Read the model definition and answer for the solid it produces. Units are mm, in the model's axes. Face numbers are marked on the shaded views. A direction names the side the tool comes from. Coordinates: 2 decimals unless noted, no trailing zeros. Loops run counter-clockwise (first coordinate to the right, second up) from the corner with the lowest first, then second, coordinate; pieces in that order, holes last.
from build123d import *

# Parameters (mm, degrees)
BOSS_EXTRUDE1_DEPTH = 7
BOSS_EXTRUDE2_DEPTH = 1
SKETCH3_W           = 57.34
SKETCH3_H           = 7
BOSS_EXTRUDE3_DEPTH = 2
SKETCH4_R           = 2
CUT_EXTRUDE1_DEPTH  = 2


with BuildPart() as part:
    # Sketch1 → Boss-Extrude1 (new body)
    with BuildSketch(Plane.XY):
        Polygon((2, -2), (-55.34, -2), (-55.34, 68.04), (-41.214427125, 68.04), (-38.674427125, 70.58), (-4.251572875, 70.58), (-1.711572875, 68.04), (2, 68.04), align=None)
        Polygon((-53.34, 0), (-53.34, 66.04), (-40.386, 66.04), (-37.846, 68.58), (-5.08, 68.58), (-2.54, 66.04), (0, 66.04), (0, 0), align=None, mode=Mode.SUBTRACT)
    extrude(amount=-BOSS_EXTRUDE1_DEPTH)

    # Sketch2 → Boss-Extrude2 (add)
    with BuildSketch(Plane(origin=(0, 0, -7), x_dir=(-1, 0, 0), z_dir=(0, 0, -1))):
        Polygon((53.34, 0), (0, 0), (0, 66.04), (2.54, 66.04), (5.08, 68.58), (37.846, 68.58), (40.386, 66.04), (53.34, 66.04), align=None)
    extrude(amount=-BOSS_EXTRUDE2_DEPTH)

    # Sketch3 → Boss-Extrude3 (add)
    with BuildSketch(Plane(origin=(0, 0, -7), x_dir=(-1, 0, 0), z_dir=(0, 0, -1))):
        with Locations((26.67, -5.5)):
            Rectangle(SKETCH3_W, SKETCH3_H)
    extrude(amount=-BOSS_EXTRUDE3_DEPTH)

    # Sketch4 → Cut-Extrude1 (cut)
    with BuildSketch(Plane.XY.offset(-5)):
        with Locations((-2.67, -5.5)):
            Circle(SKETCH4_R)
        with Locations((-50.67, -5.5)):
            Circle(SKETCH4_R)
    extrude(amount=-CUT_EXTRUDE1_DEPTH, mode=Mode.SUBTRACT)


solid = part.part
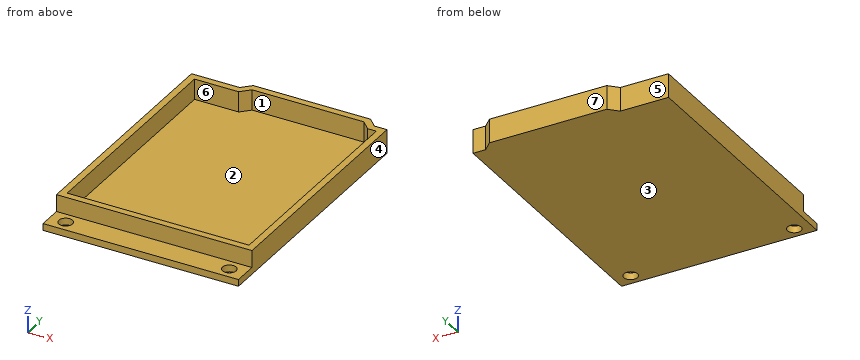
Q1. Which of the six approach directions +Z, -Z, +X, -X, +Y, -Y give full straight-line access (tool end or side, diameter ignored) to the marked faces 5, 6 and 7?
Findings below:
face 5: +Z, -Z, -X, +Y
face 6: +Z
face 7: +Z, -Z, +X, -X, +Y
Q2. A cutting plane is placed at C-C (x = -30.5). Give the vertices of the cut face in (y, z).
Findings below:
outline: (-9, -7) - (70.58, -7) - (70.58, 0) - (68.58, 0) - (68.58, -6) - (0, -6) - (0, 0) - (-2, 0) - (-2, -5) - (-9, -5) - close
Q3. A cutting plane is placed at B-B (x = -50.67). Give the vertices of the cut face in (y, z).
Findings below:
outline: (-9, -7) - (-7.5, -7) - (-7.5, -5) - (-9, -5) - close; (-3.5, -7) - (68.04, -7) - (68.04, 0) - (66.04, 0) - (66.04, -6) - (0, -6) - (0, 0) - (-2, 0) - (-2, -5) - (-3.5, -5) - close
Q4. A cutting plane is placed at A-A (y = -5.5). Give the vertices of the cut face in (x, z).
Findings below:
outline: (-55.34, -7) - (-52.67, -7) - (-52.67, -5) - (-55.34, -5) - close; (-48.67, -7) - (-4.67, -7) - (-4.67, -5) - (-48.67, -5) - close; (-0.67, -7) - (2, -7) - (2, -5) - (-0.67, -5) - close
Q5. Determine the mould class of the marked faces 1, 2, 3 and 4 for opening direction X: +X half, -X half, draft (parallel to the pull), parting line (faces both ways), or undercut.
Findings below:
face 1: undercut
face 2: undercut
face 3: draft
face 4: +X half
Q6. Straight lines are drawn through the part: probe 1 along Y at (x, z) = (-50.67, -5.7); probe 2 along Y at (x, z) = (-14.5, -2.5); probe 3 along X at (y, z) = (26, -5). For each, find the intervals that lie inside material, in ascending order.
Findings below:
probe 1: y = -9 to -7.5, -3.5 to 0, 66.04 to 68.04
probe 2: y = -2 to 0, 68.58 to 70.58
probe 3: x = -55.34 to -53.34, 0 to 2
Q7. A cutting plane is placed at D-D (y = 61.5). Give the vertices of the cut face in (x, z), then the cut area to 3 significant figures.
Findings below:
outline: (-55.34, -7) - (2, -7) - (2, 0) - (0, 0) - (0, -6) - (-53.34, -6) - (-53.34, 0) - (-55.34, 0) - close
area: 81.3 mm2
Q8. Flat-ended cylindrical pins translate along their axes: pin 1 Ø1.5 at (x, y) = (-31.5, 18.5) entering from +Z; pin 2 Ø1.5 at (x, z) = (-46, -3) entering from +Y; pin 3 Ø3 at (x, z) = (-23, -1) entering from -Y. Find the tip coordinate at first contact, or state that the pin passes through.
Findings below:
pin 1: stops at z = -6
pin 2: stops at y = 68.04
pin 3: stops at y = -2
